Input: dimensioned drawing with shaded views. Units: mm. Origin: part minimum x, y, z. A direction names the side the tool comes from. Round coordinates to 2 decimals unless told otherwise and drop trailing zeros. Order: outer loops, then holes, each group sorted by start corner. A loop starts at its lowest first (then second) coordinate and runs counter-clockwise, first axis right, second up. Notation, with made-up numbers: (5.25, -17.5) -> (30.25, -17.5) arc R33 ccw to (30.25, 11.5) -> close; hole circle Ø4 at (-26, -27). An arc over 180 degrees is marked (long way). Use a Markdown table: item, result. Add a question column.
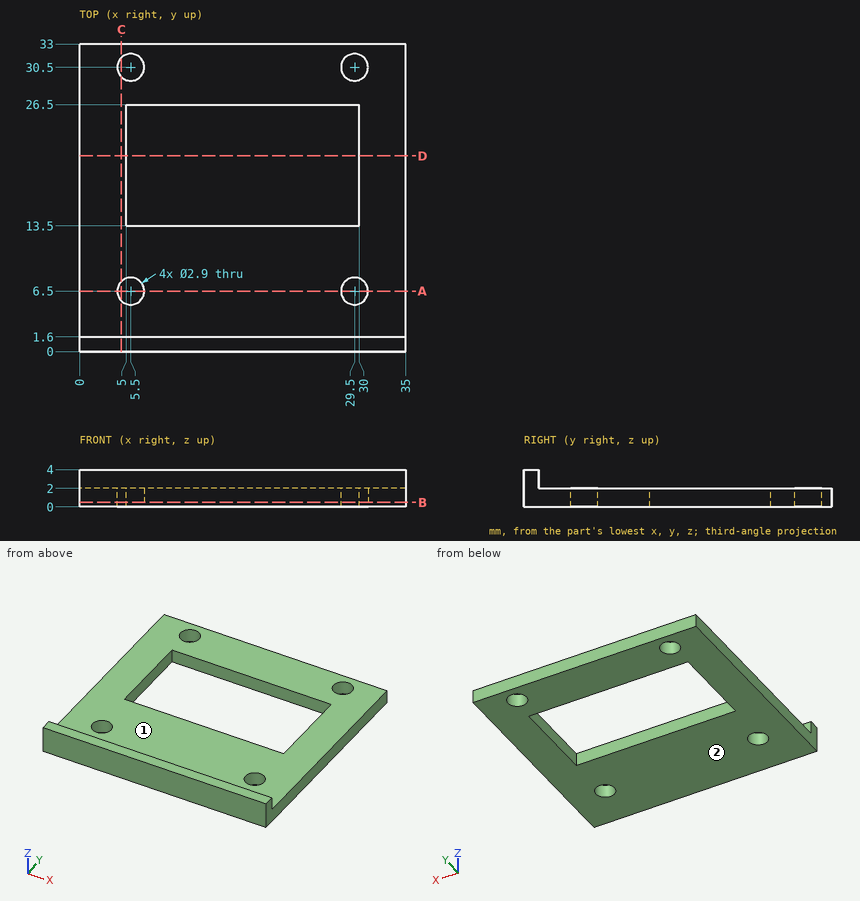
1) Line query: probe 1 along Y at (x, z) = (5.5, 1.4); probe 2 along X at (y, z) = (30, 0.55); probe 3 along Y at (x, z) = (18, 0.65). Output: solid intervals per line, ascending. Write a range as from..to.
2) First-contact query: pin 1 Ø2.5 at (x, y) = (5.5, 30.5) entering from -Z; pin 2 Ø1 at (x, z) = (10, 3) entering from +Y; pin 3 Ø8 at (x, y) = (29, 21.5) entering from +Z. Flat tips, straight axial feed; report the tip coordinate or a pass-through.
3) Reachability of the marked faces 1 and 2 from +Z, -Z, +X, -X, +Y, -Y: full face, straight path, thin tool, end or side. Return the list, or none.
4) Section B-B on z = 0.5. Output: boundary loops of the cut face in (x, y).
5) Section D-D on y = 21. Output: boundary loops of the cut face in (x, z).
6) Section C-C on x = 4.5. Output: boundary loops of the cut face in (y, z).
7) Section A-A on y = 6.5. Output: boundary loops of the cut face in (x, z).
Conclusion:
| question | item | result |
|---|---|---|
| 1 | probe 1 | y = 0..5.05, 7.95..13.5, 26.5..29.05, 31.95..33 |
| 1 | probe 2 | x = 0..4.14, 6.86..28.14, 30.86..35 |
| 1 | probe 3 | y = 0..13.5, 26.5..33 |
| 2 | pin 1 | passes through |
| 2 | pin 2 | stops at y = 1.6 |
| 2 | pin 3 | stops at z = 2 |
| 3 | face 1 | +Z, +X, -X, +Y |
| 3 | face 2 | -Z, +X, -X, +Y, -Y |
| 4 | outline | (0, 0) -> (35, 0) -> (35, 33) -> (0, 33) -> close; hole circle Ø2.9 at (5.5, 6.5); hole circle Ø2.9 at (5.5, 30.5); hole (5, 13.5) -> (30, 13.5) -> (30, 26.5) -> (5, 26.5) -> close; hole circle Ø2.9 at (29.5, 6.5); hole circle Ø2.9 at (29.5, 30.5) |
| 5 | outline | (0, 0) -> (5, 0) -> (5, 2) -> (0, 2) -> close; (30, 0) -> (35, 0) -> (35, 2) -> (30, 2) -> close |
| 6 | outline | (0, 0) -> (5.45, 0) -> (5.45, 2) -> (1.6, 2) -> (1.6, 4) -> (0, 4) -> close; (7.55, 0) -> (29.45, 0) -> (29.45, 2) -> (7.55, 2) -> close; (31.55, 0) -> (33, 0) -> (33, 2) -> (31.55, 2) -> close |
| 7 | outline | (0, 0) -> (4.05, 0) -> (4.05, 2) -> (0, 2) -> close; (6.95, 0) -> (28.05, 0) -> (28.05, 2) -> (6.95, 2) -> close; (30.95, 0) -> (35, 0) -> (35, 2) -> (30.95, 2) -> close |
